Could you check a few things on this model? Use its own coordinates, in mm. A direction names the side the tool comes from. Coordinates: 2 decimals unless noted, no trailing zeros. Write item = value, one per line. Start each with the question number.
Autodesk Inventor part; units mm, degrees
ref_plane "YZ Plane" through (0, 0, 0) normal (1, 0, 0) x (0, 1, 0)
ref_plane "XZ Plane" through (0, 0, 0) normal (0, 1, 0) x (-1, 0, 0)
ref_plane "XY Plane" through (0, 0, 0) normal (0, 0, 1) x (1, 0, 0)
sketch "Sketch1" plane through (0, 0, 0) normal (0, 1, 0) x (-1, 0, 0)
  circle A0 centre (0, 0) radius 101.6
  line L0 (101.6, -101.6) -> (101.6, 533.4)
  line L1 (101.6, 533.4) -> (-609.6, 533.4)
  line L2 (-609.6, 533.4) -> (-609.6, -101.6)
  line L3 (-609.6, -101.6) -> (101.6, -101.6)
  arc A1 (0, 381) -> (-381, 0) centre (0, 0) ccw
  line L4 (-482.6, 12.7) -> (-482.6, -101.6)
  line L5 (-381, -101.6) -> (-381, 0)
  arc A2 (0, 393.7) -> (-393.7, 0) centre (0, 0) ccw
  line L6 (-393.7, 0) -> (-393.7, -101.6)
  line L7 (0, 393.7) -> (101.6, 393.7)
  line L8 (0, 381) -> (101.6, 381)
  dimension "d0" = 203.2
  dimension "d2" = 711.2
  dimension "d5" = 279.4
  dimension "d93" = 12.7
  dimension "d104" = 635
extrude "Extrusion1" add sketch "Sketch1" along normal blind 12.7 contours L8 A1 L5 L3 L6 A2 L7 L0
sketch "Sketch5" plane through (0, 12.7, 0) normal (0, 1, 0) x (1, 0, 0)
  line L0 (393.7, 0) -> (393.7, 101.6)
  line L1 (393.7, 101.6) -> (381, 101.6)
  line L2 (381, 101.6) -> (381, 0)
  arc A0 (0, -381) -> (381, 0) centre (0, 0) ccw
  line L3 (0, -381) -> (-101.6, -381)
  line L4 (-101.6, -381) -> (-101.6, -393.7)
  circle A1 centre (-95.25, -387.35) radius 3.3782
  circle A2 centre (0, -387.35) radius 3.3782
  circle A3 centre (387.35, 0) radius 3.3782
  circle A4 centre (387.35, 95.25) radius 3.3782
  circle A5 centre (387.35, 83.3438) radius 3.3782
  circle A6 centre (387.35, 71.4375) radius 3.3782
  circle A7 centre (387.35, 59.5313) radius 3.3782
  circle A8 centre (387.35, 47.625) radius 3.3782
  circle A9 centre (387.35, 35.7188) radius 3.3782
  circle A10 centre (387.35, 23.8125) radius 3.3782
  circle A11 centre (387.35, 11.9063) radius 3.3782
  circle A12 centre (-85.725, -387.35) radius 3.3782
  circle A13 centre (-76.2, -387.35) radius 3.3782
  circle A14 centre (-66.675, -387.35) radius 3.3782
  circle A15 centre (-57.15, -387.35) radius 3.3782
  circle A16 centre (-47.625, -387.35) radius 3.3782
  circle A17 centre (-38.1, -387.35) radius 3.3782
  circle A18 centre (-28.575, -387.35) radius 3.3782
  circle A19 centre (-19.05, -387.35) radius 3.3782
  circle A20 centre (-9.525, -387.35) radius 3.3782
  circle A21 centre (10.3115, -387.2127) radius 3.3782
  circle A22 centre (20.6156, -386.801) radius 3.3782
  circle A23 centre (30.9051, -386.1151) radius 3.3782
  circle A24 centre (41.1728, -385.1556) radius 3.3782
  circle A25 centre (51.4112, -383.923) radius 3.3782
  circle A26 centre (61.6132, -382.4184) radius 3.3782
  circle A27 centre (71.7716, -380.6427) radius 3.3782
  circle A28 centre (81.8791, -378.5972) radius 3.3782
  circle A29 centre (91.9285, -376.2834) radius 3.3782
  circle A30 centre (101.9128, -373.7028) radius 3.3782
  circle A31 centre (111.8248, -370.8574) radius 3.3782
  circle A32 centre (121.6576, -367.7492) radius 3.3782
  circle A33 centre (131.4042, -364.3802) radius 3.3782
  circle A34 centre (141.0576, -360.7531) radius 3.3782
  circle A35 centre (150.611, -356.8702) radius 3.3782
  circle A36 centre (160.0577, -352.7344) radius 3.3782
  circle A37 centre (169.391, -348.3486) radius 3.3782
  circle A38 centre (178.6042, -343.7158) radius 3.3782
  circle A39 centre (187.6908, -338.8395) radius 3.3782
  circle A40 centre (196.6443, -333.723) radius 3.3782
  circle A41 centre (205.4585, -328.3699) radius 3.3782
  circle A42 centre (214.1271, -322.7841) radius 3.3782
  circle A43 centre (222.6439, -316.9696) radius 3.3782
  circle A44 centre (231.0029, -310.9304) radius 3.3782
  circle A45 centre (239.1982, -304.6707) radius 3.3782
  circle A46 centre (247.2239, -298.1952) radius 3.3782
  circle A47 centre (255.0744, -291.5083) radius 3.3782
  circle A48 centre (262.7441, -284.6148) radius 3.3782
  circle A49 centre (270.2276, -277.5195) radius 3.3782
  circle A50 centre (277.5195, -270.2276) radius 3.3782
  circle A51 centre (284.6148, -262.7441) radius 3.3782
  circle A52 centre (291.5083, -255.0744) radius 3.3782
  circle A53 centre (298.1952, -247.2239) radius 3.3782
  circle A54 centre (304.6707, -239.1982) radius 3.3782
  circle A55 centre (310.9304, -231.0029) radius 3.3782
  circle A56 centre (316.9696, -222.6439) radius 3.3782
  circle A57 centre (322.7841, -214.1271) radius 3.3782
  circle A58 centre (328.3699, -205.4585) radius 3.3782
  circle A59 centre (333.723, -196.6443) radius 3.3782
  circle A60 centre (338.8395, -187.6908) radius 3.3782
  circle A61 centre (343.7158, -178.6042) radius 3.3782
  circle A62 centre (348.3486, -169.391) radius 3.3782
  circle A63 centre (352.7344, -160.0577) radius 3.3782
  circle A64 centre (356.8702, -150.611) radius 3.3782
  circle A65 centre (360.7531, -141.0576) radius 3.3782
  circle A66 centre (364.3802, -131.4042) radius 3.3782
  circle A67 centre (367.7492, -121.6576) radius 3.3782
  circle A68 centre (370.8574, -111.8248) radius 3.3782
  circle A69 centre (373.7028, -101.9128) radius 3.3782
  circle A70 centre (376.2834, -91.9285) radius 3.3782
  circle A71 centre (378.5972, -81.8791) radius 3.3782
  circle A72 centre (380.6427, -71.7716) radius 3.3782
  circle A73 centre (382.4184, -61.6132) radius 3.3782
  circle A74 centre (383.923, -51.4112) radius 3.3782
  circle A75 centre (385.1556, -41.1728) radius 3.3782
  circle A76 centre (386.1151, -30.9051) radius 3.3782
  circle A77 centre (386.801, -20.6156) radius 3.3782
  circle A78 centre (387.2127, -10.3115) radius 3.3782
  circle A79 centre (387.35, 0) radius 3.3782
  dimension "d94" = 6.7564
  dimension "d95" = 6.35
  dimension "d96" = 6.7564
  dimension "d97" = 6.7564
  dimension "d98" = 6.35
  dimension "d99" = 6.35
  dimension "d100" = 6.35
  dimension "d101" = 6.35
  dimension "d102" = 6.35
  dimension "d103" = 101.6
  dimension "d105" = 101.6
  dimension "d108" = 11.9062
  dimension "d115" = 9.525
  dimension "d122" = 90
extrude "Extrusion5" cut sketch "Sketch5" against normal through all
sketch "Sketch11" plane through (0, 12.7, 0) normal (0, 1, 0) x (1, 0, 0)
  circle A0 centre (-19.05, -387.35) radius 3.3782
  circle A1 centre (-38.1, -387.35) radius 3.3782
  circle A2 centre (-57.15, -387.35) radius 3.3782
  circle A3 centre (-76.2, -387.35) radius 3.3782
  circle A4 centre (-95.25, -387.35) radius 3.3782
  circle A5 centre (-85.725, -387.35) radius 3.3782
  circle A6 centre (-66.675, -387.35) radius 3.3782
  circle A7 centre (-47.625, -387.35) radius 3.3782
  circle A8 centre (-28.575, -387.35) radius 3.3782
  line L0 (0, -381) -> (-101.6, -381)
  line L1 (-101.6, -381) -> (-101.6, -393.7)
  line L2 (-101.6, -393.7) -> (0, -393.7)
  line L3 (-6.35, -381) -> (-6.35, -393.7)
  dimension "d142" = 95.25
extrude "Extrusion9" cut sketch "Sketch11" against normal blind 2540
equation "\"d89\" = d46"
properties part number "Rebuild Outer Rail v1" material "Polycarbonate, Clear"
1) For P1, Ø5.5, axis at x = 373.7, z = 101.91, coming from the +Y side; P2, Ø1, axis at x = 114.5, y = 3, coming from the -Z side; P3, Ø2, axis at x = 164.5, y = 9, coming from the +Z side; P4, Ø5, axis at y = 2, z = 207.5, coming from the -X side, each with a flat end and sliding along its axis, tell me the tip position at first contact or that it passes through.
2) Suppose I cut it at A-A on y = 4.5. State how many separate pieces and enclosed holes the cut face has, plus the area to 3 significant figures.
3) Which directions (+Z, -Z, +X, -X, +Y, -Y) give clear straight access to the entire face, cutting with the end or side of a thin tool? Please do faces 1 (the flat face through (284, 12.7, 257)), 2 (the flat face through (381, 6, -52)).
4) If I drill on probe 1 along X at (y, z) = (10, 73); probe 2 along Z at (x, y) = (52, 0.5); probe 3 along Z at (x, y) = (72, 10.5) (3 decimals), over which ranges is the centre line in solid material (lowest first)? Write a range as [from, to].
Reply:
q1.P1 = through
q1.P2 = 363.23
q1.P3 = 358.14
q1.P4 = 317.9
q2.separate_pieces = 1
q2.enclosed_holes = 68
q2.area = 6,660 mm^2
q3.face_1 = +Z, -Z, +X, -X, +Y
q3.face_2 = -Z, -X, +Y, -Y
q4.probe_1 = [373.94, 377.5], [383.79, 386.87]
q4.probe_2 = [377.43, 380.6], [387.25, 390.25]
q4.probe_3 = [374.135, 377.272], [384.013, 387.06]
